Geometry: final body of the model. Coordinates: model frame, mm. Face numbers are marked on the shaded views. A direction names the side the tool comes from. Give positions to 0.01 mm unless a question says otherwise; leave off trailing zeros. Order: outer loops, then holes, each group sorted by start corner. A loop starts at its lowest first (then second) coordinate and runs counter-clockwise, first axis right, second up. Notation, with made-up numbers: (80.5, 69) -> (107.5, 69) arc R15 cw to (107.5, 76) -> close; hole circle Ø3 at (-21.5, 54). An arc over 180 degrees is marked (long way). Write item = value, one per line.
```python
from build123d import *

# Parameters (mm, degrees)
F0_W     = 80
F0_H     = 20
F1_DEPTH = 25


with BuildPart() as f1:
    # F0 (on Front) → F1 (new body)
    with BuildSketch(Plane.XZ):
        with BuildLine():
            Line((-62.5, 0), (0, 0))
            Line((0, 0), (62.5, 0))
            Line((62.5, 0), (62.5, 50))
            ThreePointArc((62.5, 50), (50.387322, 107.351956), (65.751168, 163.919758))
            ThreePointArc((65.751168, 163.919758), (0, 275), (-65.751168, 163.919758))
            ThreePointArc((-65.751168, 163.919758), (-50.387322, 107.351956), (-62.5, 50))
            Line((-62.5, 50), (-62.5, 0))
        make_face()
        with Locations((0, 35)):
            Rectangle(F0_W, F0_H, mode=Mode.SUBTRACT)
        with BuildLine():
            ThreePointArc((-25.666667, 176.204576), (0, 235), (25.666667, 176.204576))
            ThreePointArc((25.666667, 176.204576), (17.762027, 163.61574), (15, 149.009805))
            Line((15, 149.009805), (15, 100))
            ThreePointArc((15, 100), (0, 85), (-15, 100))
            Line((-15, 100), (-15, 149.009805))
            ThreePointArc((-15, 149.009805), (-17.762027, 163.61574), (-25.666667, 176.204576))
        make_face(mode=Mode.SUBTRACT)
    extrude(amount=F1_DEPTH)


solid = f1.part
```
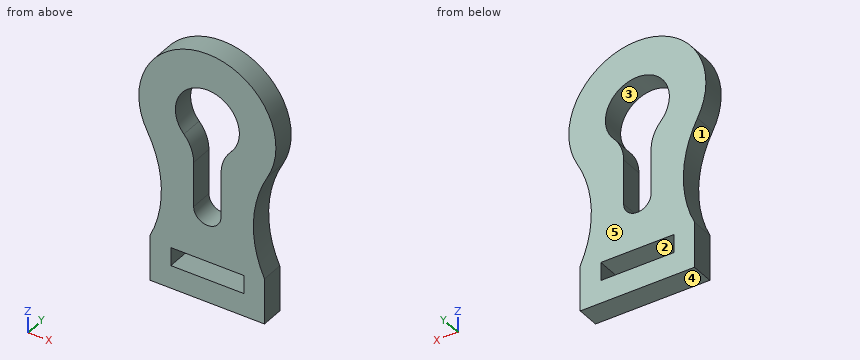
1) First-contact query: P1, Ø7.5, axis at x = -7.5, y = -17, coming from the +Z side; P2, Ø2, axis at x = -9.5, z = 90, coming from the +Y side; P3, Ø1, axis at y = -7.5, z = 176, coming from the -X side; P4, Ø10, axis at y = -11, z = 32.5, coming from the -X side. Flat tips, straight axial feed; report the tip coordinate or a pass-through.
Check sheet entries:
P1 = 274.91
P2 = through
P3 = -71.22
P4 = -62.5
2) Line query: line 1 (Z direction, x = 0, y = -14.25); line 2 (X direction, y = -12, z = 200); line 3 (Z direction, x = 3, y = -3.5). Output: solid intervals per line, ascending. Write a range as from..to.
Check sheet entries:
line_1 = 0..25, 45..85, 235..275
line_2 = -75..-35, 35..75
line_3 = 0..25, 45..85.3, 234.87..274.94
3) Reachability of the marked faces 1 and 2 from +Z, -Z, +X, -X, +Y, -Y: full face, straight path, thin tool, end or side. Return the list, or none.
Check sheet entries:
face_1 = -X, +Y, -Y
face_2 = +Y, -Y
4) Section query B-B (x = -8.5). Output: boundary loops of the cut face in (y, z), plus the area to 3 significant figures.
Check sheet entries:
outline = (-25, 0) -> (0, 0) -> (0, 25) -> (-25, 25) -> close; (-25, 45) -> (0, 45) -> (0, 87.64) -> (-25, 87.64) -> close; (-25, 233.95) -> (0, 233.95) -> (0, 274.52) -> (-25, 274.52) -> close
area = 2,710 mm²
5) Mould query, pull axis Z, two halves, no side actions, for the marked faces 3, 4 and 5. Classes: +Z half, -Z half, draft (parallel to the pull), parting line (faces both ways), or undercut.
Check sheet entries:
face_3 = undercut
face_4 = -Z half
face_5 = draft
6) Section query D-D (z = 254.5). Output: boundary loops of the cut face in (x, y).
Check sheet entries:
outline = (-51.52, -25) -> (51.52, -25) -> (51.52, 0) -> (-51.52, 0) -> close
7) Section query C-C (y = -12.5). Output: boundary loops of the cut face in (x, z).
Check sheet entries:
outline = (-65.75, 163.92) arc R125 cw to (-62.5, 50) -> (-62.5, 0) -> (62.5, 0) -> (62.5, 50) arc R125 cw to (65.75, 163.92) arc R75 ccw (long way) to start; hole (-40, 25) -> (40, 25) -> (40, 45) -> (-40, 45) -> close; hole (-25.67, 176.2) arc R40 cw to (-15, 149.01) -> (-15, 100) arc R15 ccw to (15, 100) -> (15, 149.01) arc R40 cw to (25.67, 176.2) arc R35 ccw (long way) to start
8) Section query A-A (z = 200). Output: boundary loops of the cut face in (x, y).
Check sheet entries:
outline = (-75, -25) -> (-35, -25) -> (-35, 0) -> (-75, 0) -> close; (35, -25) -> (75, -25) -> (75, 0) -> (35, 0) -> close
